```python
from build123d import *

# Parameters (mm, degrees)
SKETCH1_R           = 82.5
BOSS_EXTRUDE2_DEPTH = 50.8
SKETCH2_R           = 80
BOSS_EXTRUDE3_DEPTH = 63.5
BOSS_EXTRUDE4_START = -63.5
SKETCH3_R           = 80
BOSS_EXTRUDE4_DEPTH = 63.5
SKETCH7_R           = 79.5
CUT_EXTRUDE1_DEPTH  = 63.5
CUT_EXTRUDE2_START  = 63.5
SKETCH8_R           = 79.5
CUT_EXTRUDE2_DEPTH  = 63.5
SKETCH10_R          = 5
CUT_EXTRUDE3_DEPTH  = 63.5


with BuildPart() as part:
    # Sketch1 → Boss-Extrude2 (new body)
    with BuildSketch(Plane.XY):
        Circle(SKETCH1_R)
    extrude(amount=BOSS_EXTRUDE2_DEPTH)

    # Sketch2 → Boss-Extrude3 (add)
    with BuildSketch(Plane.XY.offset(50.8)):
        Circle(SKETCH2_R)
    extrude(amount=BOSS_EXTRUDE3_DEPTH)

    # Sketch3 → Boss-Extrude4 (add)
    with BuildSketch(Plane.XY.offset(BOSS_EXTRUDE4_START)):
        Circle(SKETCH3_R)
    extrude(amount=BOSS_EXTRUDE4_DEPTH)

    # Sketch7 → Cut-Extrude1 (cut)
    with BuildSketch(Plane.XY.offset(114.3)):
        Circle(SKETCH7_R)
    extrude(amount=-CUT_EXTRUDE1_DEPTH, mode=Mode.SUBTRACT)

    # Sketch8 → Cut-Extrude2 (cut)
    with BuildSketch(Plane.XY.offset(-63.5).offset(CUT_EXTRUDE2_START)):
        Circle(SKETCH8_R)
    extrude(amount=-CUT_EXTRUDE2_DEPTH, mode=Mode.SUBTRACT)

    # Sketch10 → Cut-Extrude3 (cut)
    with BuildSketch(Plane.XY.offset(50.8)):
        with Locations(Location((0, 74.5, 0), (0, 0, 90.000374339))):
            Circle(SKETCH10_R)
        with Locations(Location((74.5, 0, 0), (0, 0, 0.000381298))):
            Circle(SKETCH10_R)
        with Locations(Location((0, -74.5, 0), (0, 0, 270.000382713))):
            Circle(SKETCH10_R)
        with Locations(Location((-74.5, 0, 0), (0, 0, 179.999623258))):
            Circle(SKETCH10_R)
    extrude(amount=-CUT_EXTRUDE3_DEPTH, mode=Mode.SUBTRACT)


with BuildPart() as cut_extrude3_kept_piece:
    # of the separate pieces the step leaves, the one the design keeps (cut_extrude3_pieces_kept)
    add(part.part.solids().sort_by_distance((82.5, 0, 50.8))[0])


solid = cut_extrude3_kept_piece.part
```
Check sheet for the modelled part. Datum: model origin and axes. Units: mm. A direction names the side the tool comes from. Round coordinates to 2 decimals unless told otherwise and drop trailing zeros. Write each loop counter-clockwise with the first axis right and the second up, starting at its lowest first coordinate (ties: lowest second). Pieces come first, ordered by that corner, then holes. Notation, with made-up numbers: (18, -37.5) -> (59, -37.5) arc R13 cw to (59, -22.5) -> close; hole circle Ø2 at (-28.5, 36.25). An arc over 180 degrees is marked (long way). Put each result on its own line as item: value.
(1) Tool access check on faces 4 (the face through (-1, 1, 0)), 5 (the face through (-68, 43, 50.8)), 6 (the face through (-1.5, 79.27, 25.76)). Record the directions out of +Z, -Z, +X, -X, +Y, -Y that give a thin tool (end or side, any length) a straight path to the whole face; none if there is none.
Values found:
face 4: -Z
face 5: +Z
face 6: +Z, -Z
(2) Sectioned sample at C-C (z = 12.5). Enter the section's corners in (x, y), plus the area to 3 significant figures.
Values found:
outline: circle Ø165 at (0, 0); hole circle Ø10 at (-74.5, 0); hole circle Ø10 at (0, -74.5); hole circle Ø10 at (0, 74.5); hole circle Ø10 at (74.5, 0)
area: 21,100 mm^2
(3) Sectioned sample at A-A (x = 74.5). Enter the section's corners in (y, z), plus the area to 3 significant figures.
Values found:
outline: (-35.44, 0) -> (-29.15, 0) -> (-29.15, -63.5) -> (-27.75, -63.5) -> (-27.75, 0) -> (-5, 0) -> (-5, 50.8) -> (-27.75, 50.8) -> (-27.75, 114.3) -> (-29.15, 114.3) -> (-29.15, 50.8) -> (-35.44, 50.8) -> close; (5, 0) -> (27.75, 0) -> (27.75, -63.5) -> (29.15, -63.5) -> (29.15, 0) -> (35.44, 0) -> (35.44, 50.8) -> (29.15, 50.8) -> (29.15, 114.3) -> (27.75, 114.3) -> (27.75, 50.8) -> (5, 50.8) -> close
area: 3,450 mm^2
(4) Material ranges on line 1 (Y direction, x = 0, z = 20); line 2 (X direction, y = -3, z = 27.5); line 3 (Z direction, x = 52.5, y = 48.5), recorded low to high.
Values found:
line 1: y = -82.5 to -79.5, -69.5 to 69.5, 79.5 to 82.5
line 2: x = -82.45 to -78.5, -70.5 to 70.5, 78.5 to 82.45
line 3: z = 0 to 50.8
(5) Sectioned sample at D-D (y = -54). Enter the section's corners in (x, z).
Values found:
outline: (-62.37, 0) -> (-59.03, 0) -> (-59.03, -63.5) -> (-58.35, -63.5) -> (-58.35, 0) -> (58.35, 0) -> (58.35, -63.5) -> (59.03, -63.5) -> (59.03, 0) -> (62.37, 0) -> (62.37, 50.8) -> (59.03, 50.8) -> (59.03, 114.3) -> (58.35, 114.3) -> (58.35, 50.8) -> (-58.35, 50.8) -> (-58.35, 114.3) -> (-59.03, 114.3) -> (-59.03, 50.8) -> (-62.37, 50.8) -> close
(6) Mould release check, pull along X, two halves, no side actions. Record for faces 1 (the face through (-1, 1, 50.8)), 2 (the face through (-68, 43, 0)), 3 (the face through (-17.88, -80.54, 25.04)): released by +X, released by -X, zero draft, split by the parting line, or undercut.
Values found:
face 1: undercut
face 2: zero draft
face 3: split by the parting line
(7) Go/stop test with flat-tipped pins: pin 1 Ø12 at (x, z) = (64, -38.5) entering from +Y; pin 2 Ø1.5 at (x, z) = (-28.5, 2) entering from -Y; pin 3 Ø6 at (y, z) = (58, 3) entering from -X. Record where each tip stops, or that it passes through.
Values found:
pin 1: stops at y = 55.1
pin 2: stops at y = -77.69
pin 3: stops at x = -61.49
